```python
from build123d import *

# Parameters (mm, degrees)
SKETCH001_W     = 23.95
SKETCH001_H     = 20.64
SKETCH001_R     = 1.5
PAD_DEPTH       = 10
SKETCH_W        = 21.15
SKETCH_H        = 18.24
POCKET_DEPTH    = 8
SKETCH002_W     = 21.15
SKETCH002_H     = 1
PAD001_DEPTH    = 1.5
SKETCH003_W     = 21.15
SKETCH003_H     = 1
PAD002_DEPTH    = 1.5
SKETCH004_W     = 21.15
SKETCH004_H     = 0.5
PAD003_DEPTH    = 0.5
SKETCH005_W     = 21.15
SKETCH005_H     = 0.5
PAD004_DEPTH    = 0.5
SKETCH006_W     = 10
SKETCH006_H     = 6
POCKET001_DEPTH = 5


with BuildPart() as part:
    # Sketch001 → Pad (new body)
    with BuildSketch(Plane.XY):
        with Locations((0, 9.12)):
            Rectangle(SKETCH001_W, SKETCH001_H)
        with Locations((-1.5, 9.03)):
            Circle(SKETCH001_R, mode=Mode.SUBTRACT)
    extrude(amount=PAD_DEPTH)

    # Sketch → Pocket (cut)
    with BuildSketch(Plane.XY):
        with Locations((0, 9.12)):
            Rectangle(SKETCH_W, SKETCH_H)
    extrude(amount=POCKET_DEPTH, mode=Mode.SUBTRACT)

    # Sketch002 (on Face8 of Pocket) → Pad001 (join)
    with BuildSketch(Plane(origin=(0, 0, 0), x_dir=(-1, 0, 0), z_dir=(0, 1, 0))):
        with Locations((0, 4.25)):
            Rectangle(SKETCH002_W, SKETCH002_H)
    extrude(amount=PAD001_DEPTH)

    # Sketch003 (on Face10 of Pad001) → Pad002 (join)
    with BuildSketch(Plane.XZ.offset(-18.24)):
        with Locations((0, 4.25)):
            Rectangle(SKETCH003_W, SKETCH003_H)
    extrude(amount=PAD002_DEPTH)

    # Sketch004 (on Face10 of Pad002) → Pad003 (join)
    with BuildSketch(Plane.XZ.offset(-18.24)):
        with Locations((0, 1.95)):
            Rectangle(SKETCH004_W, SKETCH004_H)
    extrude(amount=PAD003_DEPTH)

    # Sketch005 (on Face8 of Pad003) → Pad004 (join)
    with BuildSketch(Plane(origin=(0, 0, 0), x_dir=(-1, 0, 0), z_dir=(0, 1, 0))):
        with Locations((0, 1.95)):
            Rectangle(SKETCH005_W, SKETCH005_H)
    extrude(amount=PAD004_DEPTH)

    # Sketch006 (on Face2 of Pad004) → Pocket001 (cut)
    with BuildSketch(Plane(origin=(-11.975, 0, 0), x_dir=(0, -1, 0), z_dir=(-1, 0, 0))):
        with Locations((-8.44, 3)):
            Rectangle(SKETCH006_W, SKETCH006_H)
    extrude(amount=-POCKET001_DEPTH, mode=Mode.SUBTRACT)


solid = part.part
```
Geometry check sheet. Reference: the model listing, model coordinates, mm. A direction names the side the tool comes from. Coordinates: 2 decimals unless noted, no trailing zeros. Order: outer loops, then holes, each group sorted by start corner. A loop starts at its lowest first (then second) coordinate and runs counter-clockwise, first axis right, second up. Notation, with made-up numbers: (74.25, 58.5) - (79.25, 58.5) arc R18 ccw to (79.25, 87.5) - close; hole circle Ø8 at (56, 34.25). An arc over 180 degrees is marked (long way). Use one line per item in the form item = value.
1. Section check C-C (x = -1.5). Record the boundary of the cut face in (y, z), then the cut area to 3 significant figures.
Here are the results:
outline = (-1.2, 0) - (0, 0) - (0, 1.7) - (0.5, 1.7) - (0.5, 2.2) - (0, 2.2) - (0, 3.75) - (1.5, 3.75) - (1.5, 4.75) - (0, 4.75) - (0, 8) - (7.53, 8) - (7.53, 10) - (-1.2, 10) - close; (10.53, 8) - (18.24, 8) - (18.24, 4.75) - (16.74, 4.75) - (16.74, 3.75) - (18.24, 3.75) - (18.24, 2.2) - (17.74, 2.2) - (17.74, 1.7) - (18.24, 1.7) - (18.24, 0) - (19.44, 0) - (19.44, 10) - (10.53, 10) - close
area = 58.0 mm²
2. Draft check along X on faces 1 (the face through (11, 8, 0)), 2 (the face through (0, 0, 1)), 3 (the face through (-11.975, 9, 7)). Enter one of: pulls with the +X half, pulls with the -X half, needs draft (parallel to the pull), parting line crosses it, or undercut.
Here are the results:
face_1 = needs draft
face_2 = undercut
face_3 = pulls with the -X half
3. Scan lines: line 1 (Y direction, x = 9, z = 4.5); line 2 (Y direction, x = -1.5, z = 8.55); line 3 (X direction, y = 3.75, z = 6.75) (3 decimals). Record each from-to range of solid material in increasing order.
Here are the results:
line_1 = -1.2 to 1.5, 16.74 to 19.44
line_2 = -1.2 to 7.53, 10.53 to 19.44
line_3 = -11.975 to -10.575, 10.575 to 11.975
4. Access from +Z, -Z, +X, -X, +Y, -Y to the whole of each face (thin tool, end or side, straight path). Record for faces 4 (the face through (0, 12, 10)), 5 (the face through (0, 19.44, 5)), 6 (the face through (0, 0, 3)), 7 (the face through (0, 16.74, 4)), 8 (the face through (-11, 9, 6)).
Here are the results:
face_4 = +Z, +X, -X, +Y, -Y
face_5 = +Z, -Z, +X, -X, +Y
face_6 = none
face_7 = -Z
face_8 = -Z, -X
5. Section check B-B (y = 9.03). Record the boundary of the cut face in (x, z) (3 decimals), then the cut area to 3 significant figures.
Here are the results:
outline = (-11.975, 6) - (-10.575, 6) - (-10.575, 8) - (-3, 8) - (-3, 10) - (-11.975, 10) - close; (0, 8) - (10.575, 8) - (10.575, 0) - (11.975, 0) - (11.975, 10) - (0, 10) - close
area = 55.9 mm²
6. Gauge pin test, flat ends, axial feed: pin 1 (0.7 mm diameter, centred on x = -11.5, y = 10, fed in from -Z); pin 2 (1.2 mm diameter, centred on x = -2, y = 17.5, fed in from -Z). Record the tip position at first contact, or that the pin passes through.
Here are the results:
pin_1 = 6
pin_2 = 1.7
7. Section check D-D (x = 1). Record the boundary of the cut face in (y, z), then the cut area to 3 significant figures.
Here are the results:
outline = (-1.2, 0) - (0, 0) - (0, 1.7) - (0.5, 1.7) - (0.5, 2.2) - (0, 2.2) - (0, 3.75) - (1.5, 3.75) - (1.5, 4.75) - (0, 4.75) - (0, 8) - (18.24, 8) - (18.24, 4.75) - (16.74, 4.75) - (16.74, 3.75) - (18.24, 3.75) - (18.24, 2.2) - (17.74, 2.2) - (17.74, 1.7) - (18.24, 1.7) - (18.24, 0) - (19.44, 0) - (19.44, 10) - (-1.2, 10) - close
area = 64.0 mm²
8. Section check A-A (y = 17.25). Record the boundary of the cut face in (x, z) (3 decimals).
Here are the results:
outline = (-11.975, 0) - (-10.575, 0) - (-10.575, 3.75) - (10.575, 3.75) - (10.575, 0) - (11.975, 0) - (11.975, 10) - (-11.975, 10) - close; hole (-10.575, 4.75) - (10.575, 4.75) - (10.575, 8) - (-10.575, 8) - close
